from build123d import *

# Parameters (mm, degrees)
SKETCH1_W           = 39.8982184
SKETCH1_H           = 5.1425094
BOSS_EXTRUDE1_DEPTH = 3.999992
BOSS_EXTRUDE2_START = -3.999992
BOSS_EXTRUDE2_DEPTH = 3.999992
CUT_EXTRUDE4_DEPTH  = 1.999996
SKETCH4_R           = 1.2494895
CUT_EXTRUDE5_DEPTH  = 22.586264202


# Read off the part's stored shape, not the designer's step: Boss-Extrude2
with BuildPart() as part:
    # Sketch1 → Boss-Extrude1 (new body)
    with BuildSketch(Plane(origin=(0, 0, 0), x_dir=(1, 0, 0), z_dir=(0, 1, 0))):
        with Locations((0, 2.5712547)):
            Rectangle(SKETCH1_W, SKETCH1_H)
    extrude(amount=BOSS_EXTRUDE1_DEPTH)

    # Boss-Extrude2 outline → Boss-Extrude2 (add)
    with BuildSketch(Plane(origin=(0, 3.999992, 0), x_dir=(1, 0, 0), z_dir=(0, 1, 0)).offset(BOSS_EXTRUDE2_START)):
        with BuildLine():
            Line((-19.809521572, 5.1425094), (-16.098890229, 5.1425094))
            ThreePointArc((-16.098890229, 5.1425094), (-16.328307217, 5.214844403), (-16.4747448, 5.405686069))
            Line((-16.4747448, 5.405686069), (-17.4189898, 7.999991269))
            Line((-17.4189898, 7.999991269), (-18.489422, 7.999991269))
            Line((-18.489422, 7.999991269), (-19.433667, 5.405686069))
            ThreePointArc((-19.433667, 5.405686069), (-19.580104584, 5.214844403), (-19.809521572, 5.1425094))
        make_face()
        with BuildLine():
            Line((-15.819722635, 5.1425094), (-12.109091292, 5.1425094))
            ThreePointArc((-12.109091292, 5.1425094), (-12.33850828, 5.214844403), (-12.484945863, 5.405686069))
            Line((-12.484945863, 5.405686069), (-13.429190863, 7.999991269))
            Line((-13.429190863, 7.999991269), (-14.499623063, 7.999991269))
            Line((-14.499623063, 7.999991269), (-15.443868063, 5.405686069))
            ThreePointArc((-15.443868063, 5.405686069), (-15.590305646, 5.214844403), (-15.819722635, 5.1425094))
        make_face()
        with BuildLine():
            Line((-11.829923697, 5.1425094), (-8.119292355, 5.1425094))
            ThreePointArc((-8.119292355, 5.1425094), (-8.348709343, 5.214844403), (-8.495146926, 5.405686069))
            Line((-8.495146926, 5.405686069), (-9.439391926, 7.999991269))
            Line((-9.439391926, 7.999991269), (-10.509824126, 7.999991269))
            Line((-10.509824126, 7.999991269), (-11.454069126, 5.405686069))
            ThreePointArc((-11.454069126, 5.405686069), (-11.600506709, 5.214844403), (-11.829923697, 5.1425094))
        make_face()
        with BuildLine():
            Line((-7.84012476, 5.1425094), (-4.129493418, 5.1425094))
            ThreePointArc((-4.129493418, 5.1425094), (-4.358910406, 5.214844403), (-4.505347989, 5.405686069))
            Line((-4.505347989, 5.405686069), (-5.449592989, 7.999991269))
            Line((-5.449592989, 7.999991269), (-6.520025189, 7.999991269))
            Line((-6.520025189, 7.999991269), (-7.464270189, 5.405686069))
            ThreePointArc((-7.464270189, 5.405686069), (-7.610707772, 5.214844403), (-7.84012476, 5.1425094))
        make_face()
        with BuildLine():
            Line((-3.850325823, 5.1425094), (-0.13969448, 5.1425094))
            ThreePointArc((-0.13969448, 5.1425094), (-0.369111469, 5.214844403), (-0.515549052, 5.405686069))
            Line((-0.515549052, 5.405686069), (-1.459794052, 7.999991269))
            Line((-1.459794052, 7.999991269), (-2.530226252, 7.999991269))
            Line((-2.530226252, 7.999991269), (-3.474471252, 5.405686069))
            ThreePointArc((-3.474471252, 5.405686069), (-3.620908835, 5.214844403), (-3.850325823, 5.1425094))
        make_face()
        with BuildLine():
            Line((0.139473114, 5.1425094), (3.850104457, 5.1425094))
            ThreePointArc((3.850104457, 5.1425094), (3.620687469, 5.214844403), (3.474249885, 5.405686069))
            Line((3.474249885, 5.405686069), (2.530004885, 7.999991269))
            Line((2.530004885, 7.999991269), (1.459572685, 7.999991269))
            Line((1.459572685, 7.999991269), (0.515327685, 5.405686069))
            ThreePointArc((0.515327685, 5.405686069), (0.368890102, 5.214844403), (0.139473114, 5.1425094))
        make_face()
        with BuildLine():
            Line((4.129272051, 5.1425094), (7.839903394, 5.1425094))
            ThreePointArc((7.839903394, 5.1425094), (7.610486406, 5.214844403), (7.464048822, 5.405686069))
            Line((7.464048822, 5.405686069), (6.519803822, 7.999991269))
            Line((6.519803822, 7.999991269), (5.449371622, 7.999991269))
            Line((5.449371622, 7.999991269), (4.505126622, 5.405686069))
            ThreePointArc((4.505126622, 5.405686069), (4.358689039, 5.214844403), (4.129272051, 5.1425094))
        make_face()
        with BuildLine():
            Line((8.119070988, 5.1425094), (11.829702331, 5.1425094))
            ThreePointArc((11.829702331, 5.1425094), (11.600285343, 5.214844403), (11.45384776, 5.405686069))
            Line((11.45384776, 5.405686069), (10.50960276, 7.999991269))
            Line((10.50960276, 7.999991269), (9.43917056, 7.999991269))
            Line((9.43917056, 7.999991269), (8.49492556, 5.405686069))
            ThreePointArc((8.49492556, 5.405686069), (8.348487976, 5.214844403), (8.119070988, 5.1425094))
        make_face()
        with BuildLine():
            Line((12.108869925, 5.1425094), (15.819501268, 5.1425094))
            ThreePointArc((15.819501268, 5.1425094), (15.59008428, 5.214844403), (15.443646697, 5.405686069))
            Line((15.443646697, 5.405686069), (14.499401697, 7.999991269))
            Line((14.499401697, 7.999991269), (13.428969497, 7.999991269))
            Line((13.428969497, 7.999991269), (12.484724497, 5.405686069))
            ThreePointArc((12.484724497, 5.405686069), (12.338286913, 5.214844403), (12.108869925, 5.1425094))
        make_face()
        with BuildLine():
            ThreePointArc((19.809300205, 5.1425094), (19.579883217, 5.214844403), (19.433445634, 5.405686069))
            Line((19.433445634, 5.405686069), (18.489200634, 7.999991269))
            Line((18.489200634, 7.999991269), (17.418768434, 7.999991269))
            Line((17.418768434, 7.999991269), (16.474523434, 5.405686069))
            ThreePointArc((16.474523434, 5.405686069), (16.328085851, 5.214844403), (16.098668862, 5.1425094))
            Line((16.098668862, 5.1425094), (19.809300205, 5.1425094))
        make_face()
    extrude(amount=BOSS_EXTRUDE2_DEPTH)

    # Sketch3 → Cut-Extrude4 (cut)
    with BuildSketch(Plane(origin=(0, 3.999992, 0), x_dir=(1, 0, 0), z_dir=(0, 1, 0))):
        Polygon((19.2496186, 2.5000077), (18.0770657, 4.530928897), (15.7319599, 4.530928897), (14.559407, 2.5000077), (15.7319599, 0.469086503), (18.0770657, 0.469086503), align=None)
        Polygon((1.7496282, 2.5000077), (0.5770753, 4.530928897), (-1.7680305, 4.530928897), (-2.9405834, 2.5000077), (-1.7680305, 0.469086503), (0.5770753, 0.469086503), align=None)
    extrude(amount=-CUT_EXTRUDE4_DEPTH, mode=Mode.SUBTRACT)

    # Sketch4 → Cut-Extrude5 (cut, through all)
    with BuildSketch(Plane(origin=(0, 1.999996, 0), x_dir=(1, 0, 0), z_dir=(0, 1, 0))):
        with Locations(Location((16.9045128, 2.5000077, 0), (0, 0, 270))):
            Circle(SKETCH4_R)
        with Locations(Location((-0.5954776, 2.5000077, 0), (0, 0, 270))):
            Circle(SKETCH4_R)
    extrude(amount=-CUT_EXTRUDE5_DEPTH, mode=Mode.SUBTRACT)


solid = part.part
The listing builds one solid part. Answer for the finished solid, in the listing's coordinates (mm). A direction names the side the tool comes from. Round coordinates to 2 decimals unless told otherwise and drop trailing zeros. Write each loop counter-clockwise with the first axis right and the second up, starting at its lowest first coordinate (ties: lowest second). Pieces come first, ordered by that corner, then holes. Notation, with made-up numbers: M -31,57.25 L -18,57.25 A34 ccw -18,91.25 Z; hole C 32,66 d7. An arc over 180 degrees is marked long. Write each question's results on one line, items separated by ' | '. Start each with the question number.
Item 1: Straight lines are drawn through the part: probe 1 along X at (y, z) = (1.15, -3.5); probe 2 along X at (y, z) = (3.25, -0.5); probe 3 along Z at (x, y) = (0, 2.7). For each, find the intervals that lie inside material, in ascending order.
Item 2: Find section B-B on x = -1. Write down the section's boundary in (y, z).
Item 3: Find section C-C on y = 2.7. Give the number of separate pieces and of enclosed holes in the cut face, and give its area (3 significant figures).
Item 4: The mould has two halves that part along X. Classify faces 4 (the flat face through (0, 2, 0)), 5 (the flat face through (-1, 3, -4.531)), 6 (the flat face through (18.97, 1.97, -6.68)), 7 (the flat face through (1.155, 3.014, -1.47)): +X half, -X half, draft (parallel to the pull), parting line (faces both ways), or undercut.
Item 5: Find section A-A on z = -2. Write down the section's boundary in (x, y), and give its area (3 significant figures).
Item 6: Which of the six approach directions +Z, -Z, +X, -X, +Y, -Y give full straight-line access (tool end or side, diameter ignored) to faces 1 (the flat face through (10, 2, -8)), 2 (the flat face through (18.655, 3.014, -1.47)), 3 (the flat face through (12.963, 1.972, -6.721))?
Answer block:
1) probe 1: x = -19.95 to -1.34, 0.15 to 16.16, 17.65 to 19.95 | probe 2: x = -19.95 to -1.79, 0.59 to 15.71, 18.09 to 19.95 | probe 3: z = -5.14 to -4.53, -0.47 to 0
2) outline: M 0,-6.74 L 4,-6.74 L 4,-4.53 L 2,-4.53 L 2,-3.68 L 0,-3.68 Z; M 0,-1.32 L 2,-1.32 L 2,-0.47 L 4,-0.47 L 4,0 L 0,0 Z
3) separate pieces: 1 | enclosed holes: 2 | area: 237 mm²
4) face 4: draft | face 5: undercut | face 6: +X half | face 7: undercut
5) outline: M -19.95,0 L -1.74,0 L -1.74,2 L -2.65,2 L -2.65,4 L -19.95,4 Z; M 0.55,0 L 15.76,0 L 15.76,2 L 14.85,2 L 14.85,4 L 1.46,4 L 1.46,2 L 0.55,2 Z; M 18.05,0 L 19.95,0 L 19.95,4 L 18.96,4 L 18.96,2 L 18.05,2 Z | area: 134 mm²
6) face 1: -Z, +X, -X, +Y, -Y | face 2: +Y | face 3: -Z, +Y, -Y
